Source: CAD feature listing. Evaluate the final solid. Frame: model axes, mm. Face numbers are marked on the shaded views. Coordinates: 2 decimals unless noted, no trailing zeros. Order: outer loops, then holes, each group sorted by start corner. A loop starts at its lowest first (then second) coordinate and runs counter-clockwise, first axis right, second up. Notation, with made-up numbers: (58.5, 45.25) -> (95.5, 45.25) arc R34 ccw to (95.5, 81.25) -> close; hole circle Ø11 at (-14, 69.25). An arc over 180 degrees is marked (long way). Put each result on its own line as item: value.
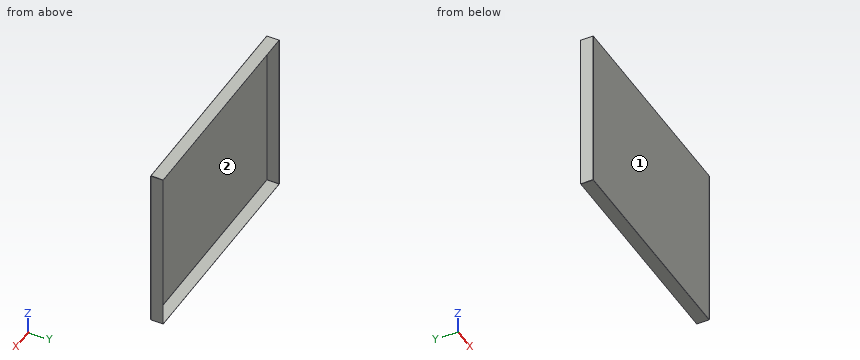
Autodesk Inventor part; units mm, degrees
ref_plane "YZ Plane" through (0, 0, 0) normal (1, 0, 0) x (0, 1, 0)
ref_plane "XZ Plane" through (0, 0, 0) normal (0, 1, 0) x (-1, 0, 0)
ref_plane "XY Plane" through (0, 0, 0) normal (0, 0, 1) x (1, 0, 0)
sketch "Sketch1" plane through (0, 0, 0) normal (0, 1, 0) x (-1, 0, 0)
  line L0 (0, 0) -> (700, 0)
  line L1 (700, 0) -> (700, -529.8)
  line L2 (700, -529.8) -> (0, -529.8)
  line L3 (0, -529.8) -> (0, 0)
  dimension "d0" = 700
  dimension "d1" = 529.8
extrude "Plate1" add sketch "Sketch1" along normal blind 0.5
sketch "Sketch2" plane through (-700, 0, -529.3) normal (0, 0, -1) x (-1, 0, 0)
  line L0 (-700, 0) -> (0, 0)
  line L1 (0, 0) -> (0, 40)
  line L2 (0, 40) -> (-700, 40)
  line L3 (-700, 40) -> (-700, 0)
edge flange "Flange1" height 40 angle 90 thickness 0.5 bend radius 0.5 thickness toward (0, 0, -1) relief tear relief width 0.5 relief depth 0.25 corner gap 0.5 corner form 2 edges at (-350, 0.5, -529.8) (0, 0.5, -264.9) (-350, 0.5, 0) (-700, 0.5, -264.9) wall of the first edge with corners at (0, 0, -529.3) (-700, 0, -529.3) (-700, 40, -529.3) (0, 40, -529.3)
bend "Bend1"
corner "Corner1"
equation "\"d3\" = BendReliefWidth"
equation "\"d4\" = BendReliefDepth"
equation "\"d5\" = MinimumRemnant"
equation "\"d6\" = BendRadius"
equation "\"d9\" = BendRadius"
equation "\"d10\" = CornerReliefSize"
equation "\"d11\" = GapSize"
equation "\"d12\" = JacobiRadiusSize"
equation "\"BendRadius\" = Thickness"
equation "\"BendReliefWidth\" = Thickness"
equation "\"BendReliefDepth\" = 0.5 * Thickness"
equation "\"CornerReliefSize\" = 4 * Thickness"
equation "\"MinimumRemnant\" = 2 * Thickness"
equation "\"TransitionRadius\" = BendRadius"
equation "\"JacobiRadiusSize\" = BendRadius"
equation "\"GapSize\" = Thickness"
equation "\"d2\" = BendRadius"
properties part number "BeddingStopper"
1. Cut plane A-A on y = 27.5. Output: boundary loops of the cut face in (x, z).
Numbers:
outline: (-700, -528.95) -> (-699.5, -528.95) -> (-699.5, -0.85) -> (-700, -0.85) -> close; (-699.15, -529.8) -> (-0.85, -529.8) -> (-0.85, -529.3) -> (-699.15, -529.3) -> close; (-699.15, -0.5) -> (-0.85, -0.5) -> (-0.85, 0) -> (-699.15, 0) -> close; (-0.5, -528.95) -> (0, -528.95) -> (0, -0.85) -> (-0.5, -0.85) -> close
2. Pull-direction query (X, two-part tool) for the marked faces 1 and 2; classes: pulls with the +X half, pulls with the -X half, needs draft (parallel to the pull), parting line crosses it, or undercut.
Numbers:
face 1: needs draft
face 2: undercut
3. Cut plane C-C on x = -455.5. Output: boundary loops of the cut face in (y, z), plus the area to 3 significant figures.
Numbers:
outline: (0, -528.8) arc R1 ccw to (1, -529.8) -> (40, -529.8) -> (40, -529.3) -> (1, -529.3) arc R0.5 cw to (0.5, -528.8) -> (0.5, -1) arc R0.5 cw to (1, -0.5) -> (40, -0.5) -> (40, 0) -> (1, 0) arc R1 ccw to (0, -1) -> close
area: 304 mm2
4. Cut plane B-B on z = -119.5. Output: boundary loops of the cut face in (x, y), plus the area to 3 significant figures.
Numbers:
outline: (-700, 1) arc R1 ccw to (-699, 0) -> (-1, 0) arc R1 ccw to (0, 1) -> (0, 40) -> (-0.5, 40) -> (-0.5, 1) arc R0.5 cw to (-1, 0.5) -> (-699, 0.5) arc R0.5 cw to (-699.5, 1) -> (-699.5, 40) -> (-700, 40) -> close
area: 389 mm2
5. First-contact query: pin 1 (1 mm diameter, centred on x = -611, y = 6, fed in from +Z); pin 2 (0.6 mm diameter, centred on y = 24.5, z = -0.5, fed in from +X); pin 3 (0.8 mm diameter, centred on y = 0.5, z = -529.5, fed in from +X); pin 4 (0.8 mm diameter, centred on x = -699.5, y = 0.5, fed in from -Z). Flat tips, straight axial feed; report the tip coordinate or a pass-through.
Numbers:
pin 1: stops at z = 0
pin 2: stops at x = -0.85
pin 3: stops at x = -1
pin 4: stops at z = -528.8
6. Ray query, line 1 along Z through (x, y) = (-359, 9.5); line 2 along X through (y, z) = (23.5, -253.5); line 3 along Y through (x, z) = (-146, -177). Return the intervals inside material, ascending.
Numbers:
line 1: z = -529.8 to -529.3, -0.5 to 0
line 2: x = -700 to -699.5, -0.5 to 0
line 3: y = 0 to 0.5
